```python
from build123d import *

# Parameters (mm, degrees)
SKETCH1_W           = 40
SKETCH1_H           = 40
BOSS_EXTRUDE1_DEPTH = 5
SKETCH2_R           = 14
SKETCH2_R_2         = 7.5
CUT_EXTRUDE1_DEPTH  = 2
CUT_EXTRUDE1_TAPER  = 30
SKETCH3_R           = 4
CUT_EXTRUDE2_DEPTH  = 6
SKETCH4_R           = 2
CUT_EXTRUDE3_DEPTH  = 6


with BuildPart() as part:
    # Sketch1 → Boss-Extrude1 (new body)
    with BuildSketch(Plane.XY):
        Rectangle(SKETCH1_W, SKETCH1_H)
    extrude(amount=BOSS_EXTRUDE1_DEPTH)

    # Sketch2 → Cut-Extrude1 (cut)
    with BuildSketch(Plane.XY.offset(5)):
        Circle(SKETCH2_R)
        Circle(SKETCH2_R_2, mode=Mode.SUBTRACT)
    extrude(amount=-CUT_EXTRUDE1_DEPTH, taper=CUT_EXTRUDE1_TAPER, mode=Mode.SUBTRACT)

    # Sketch3 → Cut-Extrude2 (cut, through all)
    with BuildSketch(Plane.XY.offset(5)):
        Circle(SKETCH3_R)
    extrude(amount=-CUT_EXTRUDE2_DEPTH, mode=Mode.SUBTRACT)

    # Sketch4 → Cut-Extrude3 (cut, through all)
    with BuildSketch(Plane.XY.offset(5)):
        with Locations((-14, 14)):
            Circle(SKETCH4_R)
        with Locations((14, 14)):
            Circle(SKETCH4_R)
        with Locations((14, -14)):
            Circle(SKETCH4_R)
        with Locations((-14, -14)):
            Circle(SKETCH4_R)
    extrude(amount=-CUT_EXTRUDE3_DEPTH, mode=Mode.SUBTRACT)


solid = part.part
```
Read the model definition and answer for the solid it produces. Units are mm, in the model's axes. A direction names the side the tool comes from. Coordinates: 2 decimals unless noted, no trailing zeros. Order: outer loops, then holes, each group sorted by start corner. A loop starts at its lowest first (then second) coordinate and runs counter-clockwise, first axis right, second up. Notation, with made-up numbers: (50.25, 29) - (99.25, 29) arc R22 ccw to (99.25, 41) - close; hole circle Ø2 at (-2.5, 69.25). An arc over 180 degrees is marked (long way). Answer as a JSON object with one key per item and string values. Group by question number.
Item 1: Section B-B (z = 0.55) is taken. Give the vertices of the cut face in (x, y).
Item 2: A flat-ended cylindrical pin translates along its axis: P1, Ø3.5, axis at x = 14, y = 14, coming from the -Z side. Find the tip coordinate at first contact, or state that the pin passes through.
Item 3: Consider probe 1 along Y at (x, z) = (-14, 2.65); probe 2 along X at (y, z) = (-12.5, 2.7); probe 3 along Y at (x, z) = (0, 2.65). Determine where each line is inside the solid, lowest interval first. Write a range as from..to.
Item 4: A tool of negligible diameter and unlimited length cuts with its end or side. For faces 4 (the face through (2.7, -8.4, 3)), 5 (the face through (12.526, 15.352, 2.535)), from which of +Z, -Z, +X, -X, +Y, -Y can it reach the whole face along a straight path? Write none if from no direction.
Item 5: Section A-A (z = 3.65) is taken. Give the vertices of the cut face in (x, y), plus the area to 3 significant figures.
Item 6: The mould has two halves that part along X. Classify faces 1 (the face through (-14, -12, 3)), 2 (the face through (-20, 0, 2)), 3 (the face through (3, -3, 5)): +X half, -X half, draft (parallel to the pull), parting line (faces both ways), or undercut.
Item 7: Section C-C (y = -15) is taken. Give the vertices of the cut face in (x, z), plus the area to 3 significant figures.
Results are:
{
 "1": {"outline": "(-20, -20) - (20, -20) - (20, 20) - (-20, 20) - close; hole circle Ø4 at (-14, -14); hole circle Ø4 at (-14, 14); hole circle Ø8 at (0, 0); hole circle Ø4 at (14, -14); hole circle Ø4 at (14, 14)"},
 "2": {"P1": "passes through"},
 "3": {"probe 1": "y = -20..-16, -12..12, 16..20", "probe 2": "x = -20..-15.32, -12.68..12.68, 15.32..20", "probe 3": "y = -20..-4, 4..20"},
 "4": {"face 4": "+Z", "face 5": "+Z, -Z"},
 "5": {"outline": "(-20, -20) - (20, -20) - (20, 20) - (-20, 20) - close; circle Ø16.56 at (0, 0); hole circle Ø4 at (-14, -14); hole circle Ø4 at (-14, 14); hole circle Ø26.44 at (0, 0); hole circle Ø8 at (0, 0); hole circle Ø4 at (14, -14); hole circle Ø4 at (14, 14)", "area": "1,170 mm^2"},
 "6": {"face 1": "undercut", "face 2": "-X half", "face 3": "draft"},
 "7": {"outline": "(-20, 0) - (-15.73, 0) - (-15.73, 5) - (-20, 5) - close; (-12.27, 0) - (12.27, 0) - (12.27, 5) - (-12.27, 5) - close; (15.73, 0) - (20, 0) - (20, 5) - (15.73, 5) - close", "area": "165 mm^2"}
}
